Model file for the job. Use its own axes, mm. A direction names the side the tool comes from. Give positions to 0.01 mm unless a question says otherwise; leave off trailing zeros. Order: outer loops, then holes, each group sorted by start corner. A loop starts at its lowest first (then second) coordinate and runs counter-clockwise, first axis right, second up. Notation, with made-up numbers: (-0.5, 49.25) -> (7.5, 49.25) arc R19 ccw to (7.5, 75.25) -> close; hole circle Ø1 at (-9.5, 53). An arc over 180 degrees is marked (long way). Use CSV: the item, a comma, the result in double quotes. Start each with the question number.
1. Wall check: line 1 (X direction, y = 36, z = -9.5); line 2 (Y direction, x = 29, z = -9.5); line 3 (Y direction, x = 30.5, z = -2.5). Give the ranges that are in metal, low to high. Write a range as from..to.
2. Cut at A-A on y = 32. List the corners of the cut face in (x, z).
3. Cut at B-B on x = 33.5. List the corners of the cut face in (y, z), then the cut area to 3 significant figures.
4. Cut at D-D on y = 5. List the corners of the cut face in (x, z).
5. Pull direction Z, two halves, no side cores. Call faces 4 (the flat face through (29, 16, 15)), 5 (the flat face through (35, 40, -10)), 6 (the flat face through (35, 35, 5)): released by +Z, released by -Z, zero draft, split by the parting line, or undercut.
6. Drop flat-ended pins along their axis: pin 1 (2 mm diameter, centred on y = 18.5, z = 12, fed in from -X); pin 2 (12 mm diameter, centred on y = 17.5, z = 10, fed in from -X); pin 3 (16 mm diameter, centred on y = 27, z = -1.5, fed in from -X). Give the stop position or say it passes through.
7. 3-axis set-ups, long thin cutter, end or side, ignore diameter. For faces 1 (the flat face through (40, 20, 0)), 2 (the flat face through (35, 30, 0)), 3 (the flat face through (25, 20, 0)): which of +Z, -Z, +X, -X, +Y, -Y reach the whole face in a straight line?
8. Cut at C-C on z = -2.75. List the corners of the cut face in (x, y).
```python
from build123d import *

# Parameters (mm, degrees)
RESSALTO_EXTRUS_O1_DEPTH = 15
ESBO_O2_W                = 10
ESBO_O2_H                = 10
CORTE_EXTRUS_O1_DEPTH    = 41


with BuildPart() as part:
    # Esboço1 → Ressalto-extrusão1 (new body, symmetric)
    with BuildSketch(Plane.XY):
        Polygon((0, 0), (20, 20), (30, 20), (30, 40), (40, 40), (40, 0), align=None)
    extrude(amount=RESSALTO_EXTRUS_O1_DEPTH, both=True)

    # Esboço2 → Corte-extrusão1 (cut, through all)
    with BuildSketch(Plane(origin=(40, 0, 0), x_dir=(0, 0, -1), z_dir=(1, 0, 0))):
        with Locations((0, 35)):
            Rectangle(ESBO_O2_W, ESBO_O2_H)
    extrude(amount=-CORTE_EXTRUS_O1_DEPTH, mode=Mode.SUBTRACT)


solid = part.part
```
Verdict:
1,line 1,"30..40"
1,line 2,"0..20"
1,line 3,"0..30"
2,outline,"(30, -15) -> (40, -15) -> (40, -5) -> (30, -5) -> close; (30, 5) -> (40, 5) -> (40, 15) -> (30, 15) -> close"
3,outline,"(0, -15) -> (40, -15) -> (40, -5) -> (30, -5) -> (30, 5) -> (40, 5) -> (40, 15) -> (0, 15) -> close"
3,area,"1,100 mm^2"
4,outline,"(5, -15) -> (40, -15) -> (40, 15) -> (5, 15) -> close"
5,face 4,"released by +Z"
5,face 5,"zero draft"
5,face 6,"undercut"
6,pin 1,"x = 17.5"
6,pin 2,"x = 11.5"
6,pin 3,"x = 19"
7,face 1,"+Z, -Z, +X, +Y, -Y"
7,face 2,"+X, -X, +Y"
7,face 3,"+Z, -Z, -X, +Y"
8,outline,"(0, 0) -> (40, 0) -> (40, 30) -> (30, 30) -> (30, 20) -> (20, 20) -> close"
